```python
from build123d import *

# Parameters (mm, degrees)
SKETCH1_R           = 3.9624
BOSS_EXTRUDE1_DEPTH = 46.355
SKETCH3_R           = 3.9624
SKETCH2_R           = 1.5875
SKETCH4_R           = 1.5875
BOSS_EXTRUDE2_DEPTH = 33.655
SKETCH5_R           = 6.477
BOSS_EXTRUDE3_DEPTH = 1.3716


with BuildPart() as part:
    # Sketch1 → Boss-Extrude1 (new body)
    with BuildSketch(Plane(origin=(0, 0, 0), x_dir=(1, 0, 0), z_dir=(0, 1, 0))):
        with Locations(Location((0, 0, 0), (0, 0, 90))):
            Circle(SKETCH1_R)
    extrude(amount=BOSS_EXTRUDE1_DEPTH)

    # Sketch3 → Loft1 section 0
    with BuildSketch(Plane(origin=(0, 46.355, 0), x_dir=(1, 0, 0), z_dir=(0, 1, 0))):
        Circle(SKETCH3_R)
    # Sketch2 → Loft1 section 1
    with BuildSketch(Plane(origin=(0, 50.165, 0), x_dir=(1, 0, 0), z_dir=(0, 1, 0))):
        Circle(SKETCH2_R)
    loft()

    # Sketch4 → Boss-Extrude2 (add)
    with BuildSketch(Plane(origin=(0, 50.165, 0), x_dir=(1, 0, 0), z_dir=(0, 1, 0))):
        with Locations(Location((0, 0, 0), (0, 0, 270))):
            Circle(SKETCH4_R)
    extrude(amount=BOSS_EXTRUDE2_DEPTH)

    # Sketch5 → Boss-Extrude3 (add)
    with BuildSketch(Plane(origin=(0, 10.16, 0), x_dir=(-1, 0, 0), z_dir=(0, -1, 0))):
        with Locations(Location((0, 0, 0), (0, 0, 90))):
            Circle(SKETCH5_R)
    extrude(amount=BOSS_EXTRUDE3_DEPTH)


solid = part.part
```
The model under review builds one solid part; all positions refer to its coordinate system, in mm. A direction names the side the tool comes from. Round coordinates to 2 decimals unless told otherwise and drop trailing zeros. Write each loop counter-clockwise with the first axis right and the second up, starting at its lowest first coordinate (ties: lowest second). Pieces come first, ordered by that corner, then holes. Notation, with made-up numbers: M -2,31.5 L 14,31.5 A21 ccw 14,66.5 Z; hole C -0.75,74.5 d7. An arc over 180 degrees is marked long. Use CSV: the item, a comma, the result in double quotes. Start each with the question number.
(1) We need section C-C, the plane z = -5.5. State the section outline as (x, y) points.
(2) We need section A-A, the plane x = 0. State the section outline as (y, z) points (1 decimal), then the cut area to 3 significant figures.
(3) For line 1 along Y through (x, z) = (-4.5, -0.75); line 2 along Y through (x, z) = (1.5, 1); line 3 along X through (y, z) = (34, 1), list the stretches that pass through material, from the lowest coordinate up.
(4) Tool access review of faces 1 (the face through (-6.323, 9.484, 1.404)), 2 (the face through (-3.93, 4.33, 0.52)), 3 (the face through (-0.966, 66.757, -1.26)): name each direction out of +Z, -Z, +X, -X, +Y, -Y from which nothing blocks a thin tool from reaching the whole face with its end or side.
(5) We need section D-D, the plane y = 20. State the section outline as (x, z) points.
(6) We need section B-B, the plane y = 66.5. State the section outline as (x, z) points (1 decimal).
(7) Clearance check with flat-ended pins moving along their axes: P1, Ø6, axis at y = 74.5, z = 2, coming from the -X side; P2, Ø5, axis at x = 4.5, z = 5, coming from the -Y side; P3, Ø5, axis at x = 2.5, y = 16.5, coming from the -Z side. State where each tip first meets the part, or that it passes through.
Findings:
1,outline,"M -3.42,8.79 L 3.42,8.79 L 3.42,10.16 L -3.42,10.16 Z"
2,outline,"M 0,-4 L 8.8,-4 L 8.8,-6.5 L 10.2,-6.5 L 10.2,-4 L 46.4,-4 L 50.2,-1.6 L 83.8,-1.6 L 83.8,1.6 L 50.2,1.6 L 46.4,4 L 10.2,4 L 10.2,6.5 L 8.8,6.5 L 8.8,4 L 0,4 Z"
2,area,"502 mm^2"
3,line 1,"8.79 to 10.16"
3,line 2,"0 to 49.82"
3,line 3,"-3.83 to 3.83"
4,face 1,"+Y, -Y"
4,face 2,"-Y"
4,face 3,"+Y"
5,outline,"C 0,0 d7.92"
6,outline,"C 0,0 d3.2"
7,P1,"x = -1.59"
7,P2,"y = 8.79"
7,P3,"z = -3.96"
